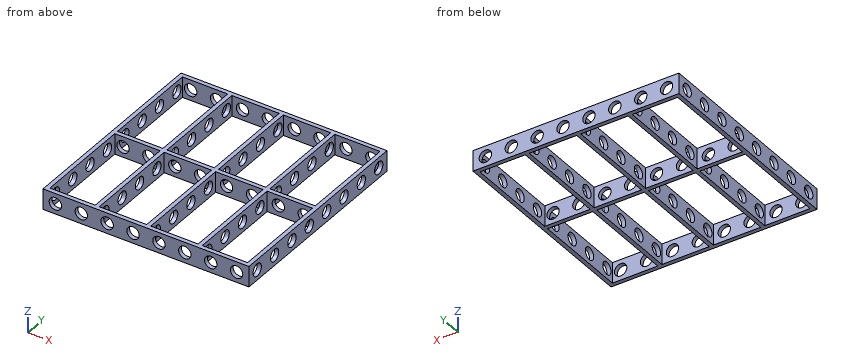
```python
from build123d import *

# Parameters (mm, degrees)
SKETCH_W               = 100
SKETCH_H               = 100
SKETCH_W_2             = 96
SKETCH_H_2             = 96
PAD_DEPTH              = 10
SKETCH001_W            = 2
SKETCH001_H            = 100
PAD001_DEPTH           = 10
LINEARPATTERN_COUNT    = 2
LINEARPATTERN_PITCH    = 25
LINEARPATTERN001_COUNT = 2
LINEARPATTERN001_PITCH = 25
SKETCH002_W            = 100
SKETCH002_H            = 2
PAD002_DEPTH           = 10
SKETCH003_R            = 3
POCKET_DEPTH           = 100.001
LINEARPATTERN002_COUNT = 8
LINEARPATTERN002_PITCH = 12.571429
SKETCH004_R            = 3
POCKET001_DEPTH        = 100.001
LINEARPATTERN003_COUNT = 8
LINEARPATTERN003_PITCH = 12.571429


with BuildPart() as part:
    # Sketch → Pad (new body)
    with BuildSketch(Plane.XY):
        Rectangle(SKETCH_W, SKETCH_H)
        Rectangle(SKETCH_W_2, SKETCH_H_2, mode=Mode.SUBTRACT)
    extrude(amount=PAD_DEPTH)

    # Sketch001 → Pad001 (join)
    with BuildSketch(Plane.XY):
        Rectangle(SKETCH001_W, SKETCH001_H)
    pad001 = extrude(amount=PAD001_DEPTH)

    # LinearPattern: Pad001 ×2
    with Locations(*[(i * LINEARPATTERN_PITCH, 0, 0) for i in range(1, LINEARPATTERN_COUNT)]):
        add(pad001)

    # LinearPattern001: Pad001 ×2
    with Locations(*[(-i * LINEARPATTERN001_PITCH, 0, 0) for i in range(1, LINEARPATTERN001_COUNT)]):
        add(pad001)

    # Sketch002 → Pad002 (join)
    with BuildSketch(Plane.XY):
        Rectangle(SKETCH002_W, SKETCH002_H)
    extrude(amount=PAD002_DEPTH)

    # Sketch003 (on Face76 of Pad002) → Pocket (cut, through all)
    with BuildSketch(Plane.YZ.offset(50)):
        with Locations((-44, 5)):
            Circle(SKETCH003_R)
    pocket = extrude(amount=-POCKET_DEPTH, mode=Mode.SUBTRACT)

    # LinearPattern002: Pocket ×8
    with Locations(*[(0, i * LINEARPATTERN002_PITCH, 0) for i in range(1, LINEARPATTERN002_COUNT)]):
        add(pocket, mode=Mode.SUBTRACT)

    # Sketch004 (on Face83 of LinearPattern002) → Pocket001 (cut, through all)
    with BuildSketch(Plane.XZ.offset(50)):
        with Locations((-44, 5)):
            Circle(SKETCH004_R)
    pocket001 = extrude(amount=-POCKET001_DEPTH, mode=Mode.SUBTRACT)

    # LinearPattern003: Pocket001 ×8
    with Locations(*[(i * LINEARPATTERN003_PITCH, 0, 0) for i in range(1, LINEARPATTERN003_COUNT)]):
        add(pocket001, mode=Mode.SUBTRACT)


solid = part.part
```
Geometry: final body of the model. Coordinates: model frame, mm. Coordinates: 2 decimals unless noted, no trailing zeros. Order: outer loops, then holes, each group sorted by start corner. A loop starts at its lowest first (then second) coordinate and runs counter-clockwise, first axis right, second up.
Item 1: Section query B-B (z = 5). State how many separate pieces and enclosed holes the cut face has, then the cut area to 3 significant figures.
Answer:
separate pieces: 57
enclosed holes: 0
area: 772 mm2
Item 2: Section query A-A (x = -44). Output: boundary loops of the cut face in (y, z).
Answer:
outline: (-50, 0) - (-48, 0) - (-48, 2) - (-50, 2) - close; (-50, 8) - (-48, 8) - (-48, 10) - (-50, 10) - close; (-1, 0) - (1, 0) - (1, 2) - (-1, 2) - close; (-1, 8) - (1, 8) - (1, 10) - (-1, 10) - close; (48, 0) - (50, 0) - (50, 2) - (48, 2) - close; (48, 8) - (50, 8) - (50, 10) - (48, 10) - close
Item 3: Section query D-D (x = -17.5). Output: boundary loops of the cut face in (y, z).
Answer:
outline: (-50, 0) - (-48, 0) - (-48, 2.32) - (-50, 2.32) - close; (-50, 7.68) - (-48, 7.68) - (-48, 10) - (-50, 10) - close; (-1, 0) - (1, 0) - (1, 2.32) - (-1, 2.32) - close; (-1, 7.68) - (1, 7.68) - (1, 10) - (-1, 10) - close; (48, 0) - (50, 0) - (50, 2.32) - (48, 2.32) - close; (48, 7.68) - (50, 7.68) - (50, 10) - (48, 10) - close
Item 4: Material intervals for line 1 along Y through (x, z) = (35, 1.5); line 2 along X through (y, z) = (12, 0.75); line 3 along Z through (x, y) = (-25.6, -44), sorted ascending.
Answer:
line 1: y = -50 to -48, -1 to 1, 48 to 50
line 2: x = -50 to -48, -26 to -24, -1 to 1, 24 to 26, 48 to 50
line 3: z = 0 to 2, 8 to 10
